```python
from build123d import *

# Parameters (mm, degrees)
BOSS_EXTRUDE1_START  = -5
SKETCH4_R            = 30
SKETCH4_R_2          = 20
BOSS_EXTRUDE1_DEPTH  = 5
SKETCH5_R            = 30
SKETCH5_R_2          = 21.75
BOSS_EXTRUDE2_DEPTH  = 15
M4_CLEARANCE_HOLE1_D = 4.3
CIRPATTERN1_COUNT    = 8


with BuildPart() as part:
    # Sketch2 → Revolve1 (revolve)
    with BuildSketch(Plane(origin=(0, 0, 0), x_dir=(0, 0, -1), z_dir=(1, 0, 0))):
        Polygon((21.328670365, 20), (21.328670365, 10.285), (0, 4.57), (-2.106039712, 4.57), (-20.171329635, 15), (-20.171329635, 20), align=None)
    revolve(axis=Axis((0, 0, 0), (0, 0, 1)))

    # Sketch4 → Boss-Extrude1 (add)
    with BuildSketch(Plane.XY.offset(20.171329635).offset(BOSS_EXTRUDE1_START)):
        Circle(SKETCH4_R)
        with Locations(Location((0, 0, 0), (0, 0, 90))):
            Circle(SKETCH4_R_2, mode=Mode.SUBTRACT)
    extrude(amount=BOSS_EXTRUDE1_DEPTH)

    # Sketch5 → Boss-Extrude2 (add)
    with BuildSketch(Plane.XY.offset(20.171329635)):
        Circle(SKETCH5_R)
        with Locations(Location((0, 0, 0), (0, 0, 270))):
            Circle(SKETCH5_R_2, mode=Mode.SUBTRACT)
    extrude(amount=BOSS_EXTRUDE2_DEPTH)

    # M4 Clearance Hole1 (through all)
    with Locations(Plane(origin=(0, 0, 15.171329635), x_dir=(-1, 0, 0), z_dir=(0, 0, -1))):
        with Locations((0, 26)):
            m4_clearance_hole1 = Hole(M4_CLEARANCE_HOLE1_D / 2)

    # CirPattern1: M4 Clearance Hole1 ×8 about axis
    cirpattern1_axis = Axis((0, 0, 0), (0, 0, 1))
    for i in range(1, CIRPATTERN1_COUNT):
        add(m4_clearance_hole1.rotate(cirpattern1_axis, i * 360 / CIRPATTERN1_COUNT), mode=Mode.SUBTRACT)


solid = part.part
```
Build history of the part. All positions in model axes, mm. A direction names the side the tool comes from. Round coordinates to 2 decimals unless told otherwise and drop trailing zeros. Write each loop counter-clockwise with the first axis right and the second up, starting at its lowest first coordinate (ties: lowest second). Pieces come first, ordered by that corner, then holes.
1) Band-saw the part on A-A, the plane x = 26. List the corners of the cut face in (y, z), and give its area (3 significant figures).
2) 3-axis set-ups, long thin cutter, end or side, ignore diameter. For faces 5 (the conical face through (6.592, -1.464, -8.145)), 6 (the flat face through (5, 15, 20.171)): which of +Z, -Z, +X, -X, +Y, -Y reach the whole face in a straight line?
3) Pin check, flat tips, straight feed: pin 1 (3 mm diameter, centred on x = -7, y = -15, fed in from +Z); pin 2 (8 mm diameter, centred on y = -19, z = -11, fed in from -X); pin 3 (5.5 mm diameter, centred on x = 18.38, y = 18.38, fed in from -Z); pin 4 (2.5 mm diameter, centred on x = 0, y = 26, fed in from +Z). Stop position of each tip, or through.
4) Band-saw the part on B-B, the plane z = 1. List the corners of the cut face in (x, y).
5) Mould opens along X. For faces 1 (the cylindrical face through (21.565, 2.831, 27.566)), 2 (the flat face through (-0.4, 20.4, 15.171)), 3 (the cylindrical face through (-17.738, -16.335, 25.311)), 4 (the cylindrical face through (19.524, -4.336, -3.334)) say: +X half, -X half, draft (parallel to the pull), parting line (faces both ways), or undercut.
6) Band-saw the part on D-D, the plane z = 29. Give the number of separate pieces and of enclosed holes in the cut face, and give its area (3 significant figures).
7) Drill centre lines: probe 1 along Y at (x, z) = (0, 1); probe 2 along X at (y, z) = (-0.5, 15.5); probe 3 along Z at (x, y) = (21, 6.5). Where is each one in solid material? Low to high.
Ans:
1. outline: (-14.97, 15.17) - (-2.15, 15.17) - (-2.15, 35.17) - (-14.97, 35.17) - close; (2.15, 15.17) - (14.97, 15.17) - (14.97, 35.17) - (2.15, 35.17) - close
1. area: 513 mm2
2. face 5: -Z
2. face 6: +Z
3. pin 1: stops at z = 20.17
3. pin 2: stops at x = -13.23
3. pin 3: stops at z = 15.17
3. pin 4: passes through
4. outline: circle Ø40 at (0, 0); hole circle Ø9.14 at (0, 0)
5. face 1: undercut
5. face 2: draft
5. face 3: undercut
5. face 4: parting line
6. separate pieces: 1
6. enclosed holes: 9
6. area: 1,230 mm2
7. probe 1: y = -20 to -4.57, 4.57 to 20
7. probe 2: x = -30 to -28.09, -23.91 to -12.29, 12.29 to 23.91, 28.09 to 30
7. probe 3: z = 15.17 to 35.17
